Verification items for this drawing (mm, ordinates from the low corner). A direction names the side the tool comes from. Round coordinates to 2 decimals unless told otherwise and drop trailing zeros. Loops run counter-clockwise (first coordinate to the right, second up) from the corner with the lowest first, then second, coordinate; pieces in that order, holes last. Notation, with made-up numbers: M 58,37 L 103,37 A28 ccw 103,56 Z; hole C -22,0.5 d1. An arc over 180 degrees is marked long. Use one line per item in the form item = value. Start each with the question number.
1. Go/stop test with flat-tipped pins: pin 1 (5 mm diameter, centred on x = 8, y = 2.5, fed in from +Z); pin 2 (2 mm diameter, centred on y = 9, z = 24.1, fed in from +X). Record where each tip stops, or that it passes through.
2. Cross-section at B-B (y = 9). Record the boundary of the cut face in (x, z), then the cut area to 3 significant figures.
3. Cross-section at D-D (z = 24.1). Record the boundary of the cut face in (x, y), then the cut area to 3 significant figures.
4. Draft check along Y on the marked faces 4, 5 and 6. Enter one of: pulls with the +Y half, pulls with the -Y half, needs draft (parallel to the pull), parting line crosses it, or undercut.
5. Set-up check for the marked faces 1, 2 and 3: record each of +Z, -Z, +X, -X, +Y, -Y from which the full face is reachable in a straight line by a thin tool's end or side.
6. Material ranges on line 1 (X direction, y = 7, z = 4); line 2 (X direction, y = 16.25, z = 13.75); line 3 (Y direction, x = 12.5, z = 1.5), recorded low to high.
7. Cross-section at A-A (x = 12.45). Record the boundary of the cut face in (y, z), then the cut area to 3 significant figures.
8. Cross-section at C-C (z = 19.5). Record the boundary of the cut face in (x, y).
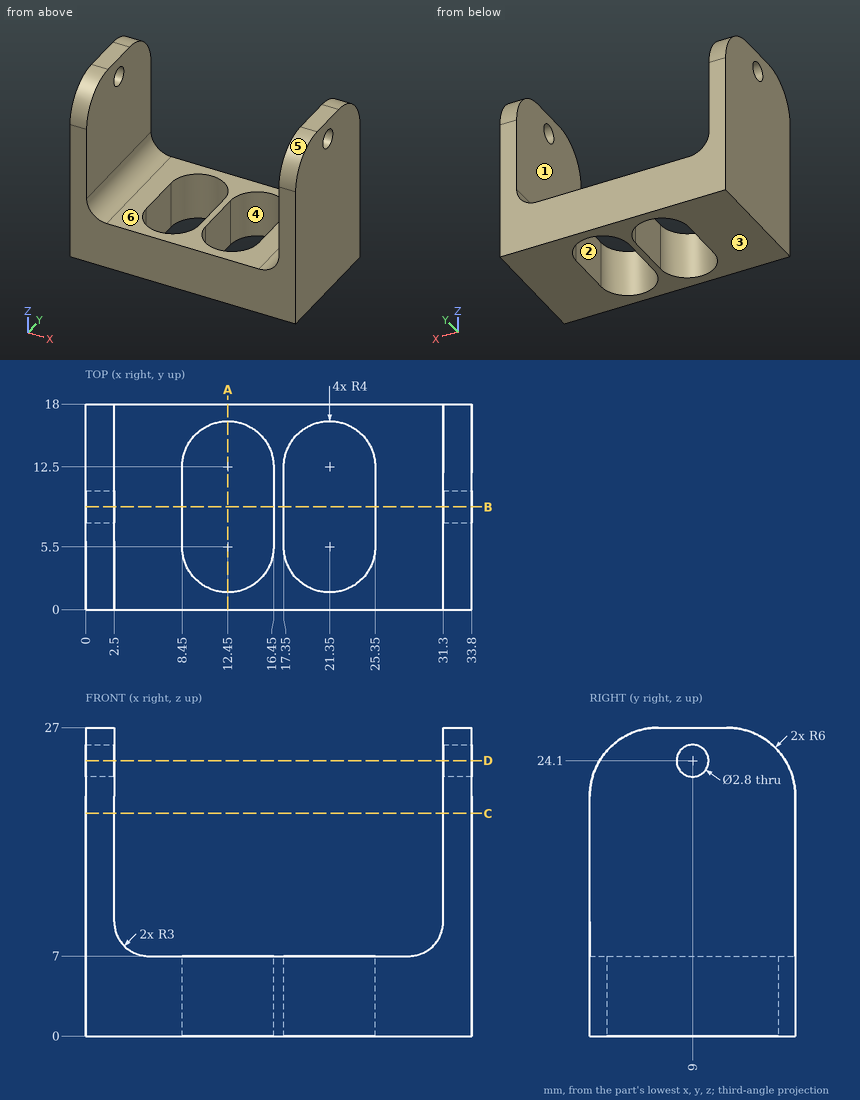
Reported:
q1.pin_1 = 7
q1.pin_2 = through
q2.outline = M 0,0 L 8.45,0 L 8.45,7 L 5.5,7 A3 cw 2.5,10 L 2.5,22.7 L 0,22.7 Z; M 0,25.5 L 2.5,25.5 L 2.5,27 L 0,27 Z; M 16.45,0 L 17.35,0 L 17.35,7 L 16.45,7 Z; M 25.35,0 L 33.8,0 L 33.8,22.7 L 31.3,22.7 L 31.3,10 A3 cw 28.3,7 L 25.35,7 Z; M 31.3,25.5 L 33.8,25.5 L 33.8,27 L 31.3,27 Z
q2.area = 214 mm²
q3.outline = M 0,0.86 L 2.5,0.86 L 2.5,7.6 L 0,7.6 Z; M 0,10.4 L 2.5,10.4 L 2.5,17.14 L 0,17.14 Z; M 31.3,0.86 L 33.8,0.86 L 33.8,7.6 L 31.3,7.6 Z; M 31.3,10.4 L 33.8,10.4 L 33.8,17.14 L 31.3,17.14 Z
q3.area = 67.4 mm²
q4.face_4 = undercut
q4.face_5 = pulls with the -Y half
q4.face_6 = needs draft
q5.face_1 = +Z, +Y, -Y
q5.face_2 = +Z, -Z
q5.face_3 = -Z, +X, -X, +Y, -Y
q6.line_1 = 0 to 8.45, 16.45 to 17.35, 25.35 to 33.8
q6.line_2 = 0 to 2.5, 31.3 to 33.8
q6.line_3 = 0 to 1.5, 16.5 to 18
q7.outline = M 0,0 L 1.5,0 L 1.5,7 L 0,7 Z; M 16.5,0 L 18,0 L 18,7 L 16.5,7 Z
q7.area = 21.0 mm²
q8.outline = M 0,0 L 2.5,0 L 2.5,18 L 0,18 Z; M 31.3,0 L 33.8,0 L 33.8,18 L 31.3,18 Z
